from build123d import *
from build123d.topology import SkipClean

# Parameters (mm, degrees)
BOSS_EXTRU_1_DEPTH      = 25.4
BOSS_EXTRU_3_DEPTH      = 25.4
BOSS_EXTRU_3_DEPTH_BACK = 50.8
ESQUISSE4_R             = 3.175
ENL_V_MAT_EXTRU_2_DEPTH = 181.045576616


with BuildPart() as part:
    # Esquisse1 → Boss.-Extru.1 (new body)
    with BuildSketch(Plane(origin=(0, 0, 0), x_dir=(1, 0, 0), z_dir=(0, 1, 0))):
        with BuildLine():
            Line((-86.988995356, -59.030471555), (-106.422794534, -50.551910349))
            ThreePointArc((-106.422794534, -50.551910349), (-109.945906268, -42.346245775), (-112.837401426, -33.897310746))
            ThreePointArc((-112.837401426, -33.897310746), (-115.930942089, -21.007701033), (-117.557008422, -7.852172131))
            ThreePointArc((-117.557008422, -7.852172131), (-117.13621005, -5.119362004), (-115.593885954, -2.824463565))
            ThreePointArc((-115.593885954, -2.824463565), (-97.983870719, 11.30660622), (-78.273017823, 22.319419119))
            ThreePointArc((-78.273017823, 22.319419119), (-74.924997914, 21.864997198), (-73.882142487, 18.651247184))
            ThreePointArc((-73.882142487, 18.651247184), (-68.674121781, -33.019766772), (-31.56784929, -69.353521116))
            Line((-31.56784929, -69.353521116), (-12.068063318, -77.860870983))
            ThreePointArc((-12.068063318, -77.860870983), (1.055821232, -111.298628897), (-32.381936682, -124.422513448))
            Line((-32.381936682, -124.422513448), (-96.139091412, -96.606596769))
            ThreePointArc((-96.139091412, -96.606596769), (-97.611067531, -95.297834712), (-98.027929733, -93.37278985))
            ThreePointArc((-98.027929733, -93.37278985), (-95.927030568, -81.790963802), (-92.067463697, -70.670882171))
            Line((-92.067463697, -70.670882171), (-86.988995356, -59.030471555))
        make_face()
    extrude(amount=BOSS_EXTRU_1_DEPTH)

    # Esquisse2 → Boss.-Extru.3 (add, two sides: drawn at the far end of the back side and taken through both)
    with SkipClean():  # the faces are left unmerged after this step: merging them gives an invalid solid
        with BuildSketch(Plane(origin=(0, 25.4, 0), x_dir=(1, 0, 0), z_dir=(0, 1, 0)).offset(-BOSS_EXTRU_3_DEPTH_BACK)):
            with BuildLine():
                Line((-12.068063318, -77.860870983), (-31.56784929, -69.353521116))
                ThreePointArc((-31.56784929, -69.353521116), (-68.674121781, -33.019766772), (-73.882142487, 18.651247184))
                ThreePointArc((-73.882142487, 18.651247184), (-76.183429791, 22.506805087), (-80.038987694, 20.205517783))
                ThreePointArc((-80.038987694, 20.205517783), (-74.38590155, -35.794415076), (-34.152036158, -75.1541145))
                Line((-34.152036158, -75.1541145), (-14.607297489, -83.681076291))
                ThreePointArc((-14.607297489, -83.681076291), (-10.42757775, -82.040590723), (-12.068063318, -77.860870983))
            make_face()
        extrude(amount=BOSS_EXTRU_3_DEPTH + BOSS_EXTRU_3_DEPTH_BACK)
    add(part.part.scale(1), mode=Mode.REPLACE)  # the faces are merged on a copy

    # Esquisse4 → Enl_v. mat.-Extru.2 (cut, through all)
    with BuildSketch(Plane(origin=(0, 25.4, 0), x_dir=(1, 0, 0), z_dir=(0, 1, 0))):
        with Locations(Location((-22.225, -101.141692216, 0), (0, 0, 270))):
            Circle(ESQUISSE4_R)
    extrude(amount=-ENL_V_MAT_EXTRU_2_DEPTH, mode=Mode.SUBTRACT)


solid = part.part
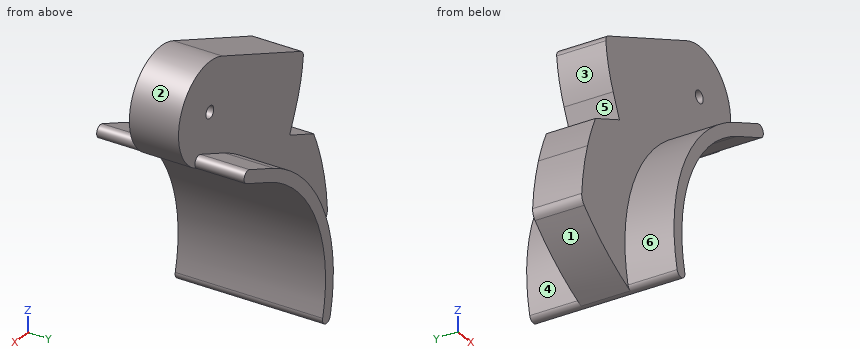
Source: CAD feature listing. Evaluate the final solid. Frame: model axes, mm. Face numbers are marked on the shaded views. A direction names the side the tool comes from. Round coordinates to 2 decimals unless told otherwise and drop trailing zeros. Loops run counter-clockwise (first coordinate to the right, second up) from the corner with the lowest first, then second, coordinate; pieces in that order, holes last.
Q1. Section B-B, the plane z = 43.5. Return loops of the section in (x, y), plus the area to 3 significant figures.
Q2. Section C-C, the plane x = -53.5. Return loops of the section in (y, z).
Q3. Mould query, pull axis Z, two halves, no side actions, for the marked faces 1, 2 and 3. Classes: pulls with the +Z half, pulls with the -Z half, needs draft (parallel to the pull), parting line crosses it, or undercut.
Q4. Access query for the marked faces 4, 5 and 6. Directions: +Z, -Z, +X, -X, +Y, -Y. A direction counts if a zero-diameter tool reaches every point of the face in a straight line with its end or side. Return the directions, or none.
Q5. Ray query, line 1 (Y direction, x = -85, z = 42.5); line 2 (X direction, y = 20.5, z = 99.5); line 3 (Z direction, x = -107.5, y = 1). Return the intervals inside material, ascending.
Q6. Section D-D, the plane y = -12. Return loops of the section in (x, z) (3 decimals), plus the area to 3 significant figures.
Q7. First-contact query: P1, Ø1.5, axis at x = -39.5, y = 1, coming from the +Z side; P2, Ø1, axis at x = -18, y = 23.5, coming from the +Z side; P3, Ø2, axis at y = -5.5, z = 33.5, coming from the +X side. Flat tips, straight axial feed; report the tip coordinate or a pass-through.
Solutions:
1. outline: (-109.49, 0) - (-70.16, 0) - (-70.16, -25.4) - (-62.56, -25.4) - (-62.56, 50.8) - (-70.16, 50.8) - (-70.16, 25.4) - (-109.49, 25.4) - close
1. area: 1,580 mm2
2. outline: (-25.4, 54.26) - (50.8, 54.26) - (50.8, 62.87) - (25.4, 62.87) - (25.4, 115.21) - (0, 115.21) - (0, 62.87) - (-25.4, 62.87) - close
3. face 1: pulls with the -Z half
3. face 2: parting line crosses it
3. face 3: undercut
4. face 4: -X, +Y
4. face 5: -X, +Y, -Y
4. face 6: -X, -Y
5. line 1: y = 0 to 25.4
5. line 2: x = -89.51 to -24.94, -19.51 to 3.12
5. line 3: z = -4.27 to 48.22
6. outline: (-80.039, -20.206) arc R3.175 ccw to (-73.882, -18.651) arc R76.2 cw to (-31.568, 69.354) - (-12.068, 77.861) arc R3.175 ccw to (-14.607, 83.681) - (-34.152, 75.154) arc R82.55 ccw to start
6. area: 868 mm2
7. P1: stops at z = 121.64
7. P2: stops at z = 126.27
7. P3: stops at x = -67.94
